from build123d import *

# Parameters (mm, degrees)
EXTRUDE_1_DEPTH   = 2
HOLE_WIZARD_M81_D = 9
CHAMFER_1_SIZE    = 2.5


with BuildPart() as part:
    # Эскиз3 → Бобышка-Вытянуть1 (new body)
    with BuildSketch(Plane(origin=(0, 0, 0), x_dir=(1, 0, 0), z_dir=(0, 0, -1))):
        Polygon((0, 0), (100, 0), (100, 100), (75, 143.301270189), (0, 100), align=None)
    extrude(amount=EXTRUDE_1_DEPTH)

    # Отверстие с зазором M81 (through all)
    with Locations(Plane(origin=(0, 0, -2), x_dir=(1, 0, 0), z_dir=(0, 0, -1))):
        with Locations((25, 25), (75, 25), (21.650635095, 83.632486541), (65.849364905, 109.150635095)):
            Hole(HOLE_WIZARD_M81_D / 2)

    # Фаска1
    chamfer_1_edges = [part.edges().sort_by_distance(p)[0] for p in [
        (75, -143.301270189, -1),
        (100, 0, -1),
        (0, 0, -1),
    ]]
    chamfer(chamfer_1_edges, length=CHAMFER_1_SIZE)


solid = part.part
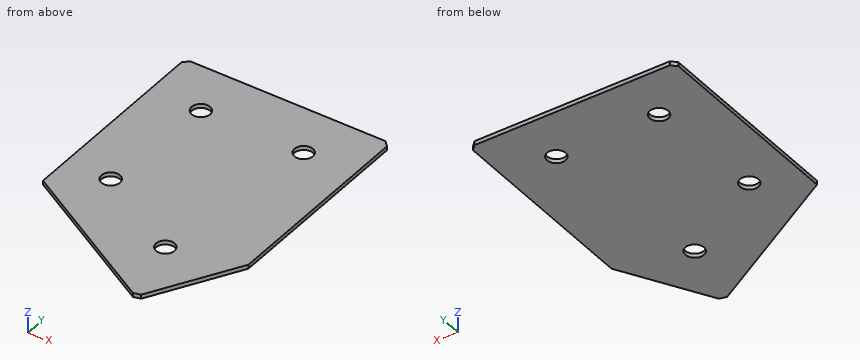
Here's how the part is built. I have some questions about the finished solid (model axes, mm). Give positions to 0.01 mm unless a question says otherwise; leave off trailing zeros. Write each loop counter-clockwise with the first axis right and the second up, starting at its lowest first coordinate (ties: lowest second). Pieces come first, ordered by that corner, then holes. Notation, with made-up numbers: (-20, -33.75) -> (12, -33.75) arc R21 ccw to (12, -7.75) -> close; hole circle Ø8 at (41.25, -16). An arc over 180 degrees is marked (long way). Use one line per item in the form item = value. Start each with the question number.
1. Imagine slicing it at D-D on z = -1.35. List the corners of the cut face in (x, y) for me.
2. Imagine slicing it at C-C on y = -111.5. List the corners of the cut face in (x, z) for me, plus the area to 3 significant figures.
3. If I drill on L1, parallel to X at y = -27.5, z = -1.55; L2, parallel to X at y = -25, z = -0.75; L3, parallel to Y at x = 25, z = -1.5, over which ranges is the centre line in solid material (lowest first)?
4. Will these pins go through, and if not, where does the flat tip stop? pin 1 Ø1 at (x, y) = (63.5, -14.5) entering from +Z; pin 2 Ø8 at (x, y) = (25, -25) entering from +Z.
5. Imagine slicing it at B-B on x = 28. List the corners of the cut face in (y, z) for me, plus the area to 3 significant figures.
6. Imagine slicing it at A-A on y = -25. List the corners of the cut face in (x, z) for me.
Entries:
q1.outline = (0, -100) -> (72.83, -142.05) -> (76.25, -141.14) -> (100, -100) -> (100, -2.5) -> (97.5, 0) -> (2.5, 0) -> (0, -2.5) -> close; hole circle Ø9 at (21.65, -83.63); hole circle Ø9 at (25, -25); hole circle Ø9 at (65.85, -109.15); hole circle Ø9 at (75, -25)
q2.outline = (19.92, -2) -> (62.01, -2) -> (62.01, 0) -> (19.92, 0) -> close; (69.69, -2) -> (93.36, -2) -> (93.36, 0) -> (69.69, 0) -> close
q2.area = 132 mm²
q3.L1 = 0 to 21.26, 28.74 to 71.26, 78.74 to 100
q3.L2 = 0 to 20.5, 29.5 to 70.5, 79.5 to 100
q3.L3 = -114.43 to -86.64, -80.63 to -29.5, -20.5 to 0
q4.pin_1 = 0
q4.pin_2 = through
q5.outline = (-116.17, -2) -> (-28.35, -2) -> (-28.35, 0) -> (-116.17, 0) -> close; (-21.65, -2) -> (0, -2) -> (0, 0) -> (-21.65, 0) -> close
q5.area = 219 mm²
q6.outline = (0, -2) -> (20.5, -2) -> (20.5, 0) -> (0, 0) -> close; (29.5, -2) -> (70.5, -2) -> (70.5, 0) -> (29.5, 0) -> close; (79.5, -2) -> (100, -2) -> (100, 0) -> (79.5, 0) -> close
